from build123d import *

# Parameters (mm, degrees)
SKETCH_W     = 348
SKETCH_H     = 475
PAD_DEPTH    = 8
CHAMFER_SIZE = 4


with BuildPart() as part:
    # Sketch → Pad (new body)
    with BuildSketch(Plane.XZ):
        with Locations((-36.713229, -51.613825)):
            Rectangle(SKETCH_W, SKETCH_H)
    extrude(amount=PAD_DEPTH)

    # Chamfer
    chamfer_edges = [part.edges().sort_by_distance(p)[0] for p in [
        (-36.713229, -8, -289.113825),
        (137.286771, -8, -51.613825),
        (-36.713229, -8, 185.886175),
        (-210.713229, -8, -51.613825),
    ]]
    chamfer(chamfer_edges, length=CHAMFER_SIZE)


solid = part.part
Could you check a few things on this model? Use its own coordinates, in mm. Coordinates: 2 decimals unless noted, no trailing zeros. Loops run counter-clockwise (first coordinate to the right, second up) from the corner with the lowest first, then second, coordinate; pieces in that order, holes last. Notation, with made-up numbers: (-9, 52) -> (43, 52) arc R12 cw to (43, 63) -> close; hole circle Ø6 at (18, 76.25). An arc over 180 degrees is marked (long way). Answer in a Markdown table with one row per item.
(1) Imagine slicing it at A-A (y = -6.5). List the corners of the cut face in (x, z) for me, plus the area to 3 significant figures.
Results found:
| item | result |
|---|---|
| outline | (-208.21, -286.61) -> (134.79, -286.61) -> (134.79, 183.39) -> (-208.21, 183.39) -> close |
| area | 161,000 mm^2 |
(2) Thinking about a two-plate mould opening in Y: for faces 1 (the face through (-39, -8, -48)), 2 (the face through (-39, 0, -48)), which applies, released by +Y, released by -Y, zero draft, split by the parting line, or undercut?
Results found:
| item | result |
|---|---|
| face 1 | released by -Y |
| face 2 | released by +Y |
(3) If I drill on probe 1 along Z at (x, y) = (24.5, -6); probe 2 along X at (y, z) = (-6.75, -132); probe 3 along Z at (x, y) = (-163.5, -4.25), over which ranges is the centre line in solid material (lowest first)?
Results found:
| item | result |
|---|---|
| probe 1 | z = -287.11 to 183.89 |
| probe 2 | x = -207.96 to 134.54 |
| probe 3 | z = -288.86 to 185.64 |
(4) Will these pins go through, and if not, where does the flat tip stop? pin 1 Ø1.5 at (y, z) = (-7, -144) entering from -X; pin 2 Ø1 at (x, z) = (43.5, 127) entering from +Y.
Results found:
| item | result |
|---|---|
| pin 1 | stops at x = -208.46 |
| pin 2 | stops at y = 0 |
